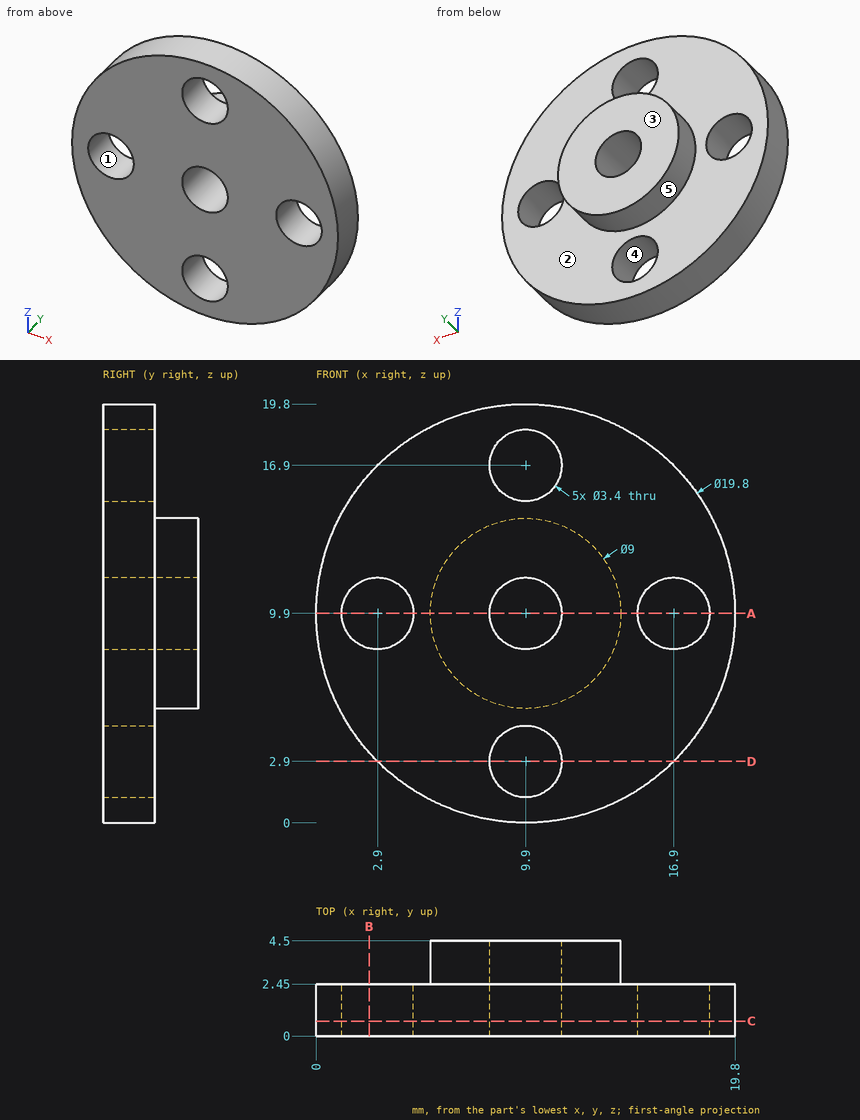
Verification items for this drawing (mm, ordinates from the low corner). A direction names the side the tool comes from. Coordinates: 2 decimals unless noted, no trailing zeros. Order: outer loops, then holes, each group sorted by start corner. A loop starts at its lowest first (then second) coordinate and runs counter-clockwise, first axis right, second up. Notation, with made-up numbers: M -22,73.5 L 25,73.5 A23 ccw 25,85.5 Z; hole C -30,83 d1. An arc over 180 degrees is marked long. Write each question's results on one line, items separated by ' | '.
1) Access from +Z, -Z, +X, -X, +Y, -Y to the whole of each face (thin tool, end or side, straight path). Record for the marked faces 1 and 2.
Solved:
face 1: +Y, -Y | face 2: +Y
2) Section check C-C on y = 0.7. Record the cut outline in (x, z), plus the area to 3 significant figures.
Solved:
outline: C 9.9,9.9 d19.8; hole C 2.9,9.9 d3.4; hole C 9.9,2.9 d3.4; hole C 9.9,9.9 d3.4; hole C 9.9,16.9 d3.4; hole C 16.9,9.9 d3.4 | area: 263 mm²
3) Section check B-B on x = 2.5. Record the cut outline in (y, z), plus the area to 3 significant figures.
Solved:
outline: M 0,3.32 L 2.45,3.32 L 2.45,8.25 L 0,8.25 Z; M 0,11.55 L 2.45,11.55 L 2.45,16.48 L 0,16.48 Z | area: 24.1 mm²
4) Gauge pin test, flat end, axial feed: pin 1 Ø1 at (x, z) = (12, 14.5) entering from +Y. Record the tip position at first contact, or that the pin passes through.
Solved:
pin 1: stops at y = 2.45
5) Section check A-A on z = 9.9. Record the cut outline in (x, y), plus the area to 3 significant figures.
Solved:
outline: M 0,0 L 1.2,0 L 1.2,2.45 L 0,2.45 Z; M 4.6,0 L 8.2,0 L 8.2,4.5 L 5.4,4.5 L 5.4,2.45 L 4.6,2.45 Z; M 11.6,0 L 15.2,0 L 15.2,2.45 L 14.4,2.45 L 14.4,4.5 L 11.6,4.5 Z; M 18.6,0 L 19.8,0 L 19.8,2.45 L 18.6,2.45 Z | area: 35.0 mm²
6) Release check for a two-part mould opening along Z. For the marked faces 3, 4 and 5 record: pulls with the +Z half, pulls with the -Z half, needs draft (parallel to the pull), parting line crosses it, or undercut.
Solved:
face 3: needs draft | face 4: undercut | face 5: parting line crosses it
7) Section check D-D on z = 2.9. Record the cut outline in (x, y), plus the area to 3 significant figures.
Solved:
outline: M 2.9,0 L 8.2,0 L 8.2,2.45 L 2.9,2.45 Z; M 11.6,0 L 16.9,0 L 16.9,2.45 L 11.6,2.45 Z | area: 26.0 mm²
8) Scan lines: line 1 along X through (y, z) = (0.5, 10); line 2 along X through (y, z) = (0.9, 10.5). Record each from-to range of solid material in increasing order. Write a range as [from, to].
Solved:
line 1: x = [0, 1.2], [4.6, 8.2], [11.6, 15.2], [18.6, 19.8] | line 2: x = [0.02, 1.31], [4.49, 8.31], [11.49, 15.31], [18.49, 19.78]
